from build123d import *

# Parameters (mm, degrees)
RECTANGLE127_AS_DRAWN_W                      = 25
RECTANGLE127_AS_DRAWN_H                      = 3
EXTRUDE155_DEPTH                             = 3
EXTRUDE155_ONTO_RECTANGLE127_ROLL_ANGLE      = -90
EXTRUDE155_ONTO_RECTANGLE127_PLACEMENT_ANGLE = 180
RECTANGLE128_AS_DRAWN_W                      = 25
RECTANGLE128_AS_DRAWN_H                      = 3
EXTRUDE157_DEPTH                             = 3
EXTRUDE157_ONTO_RECTANGLE128_ROLL_ANGLE      = -90
EXTRUDE157_ONTO_RECTANGLE128_PLACEMENT_ANGLE = 180
RECTANGLE130_AS_DRAWN_W                      = 25
RECTANGLE130_AS_DRAWN_H                      = 3
EXTRUDE162_DEPTH                             = 3
EXTRUDE162_ONTO_RECTANGLE130_ROLL_ANGLE      = -90
EXTRUDE162_ONTO_RECTANGLE130_PLACEMENT_ANGLE = 180
EXTRUDE160_DEPTH                             = 3
EXTRUDE160_ONTO_RECTANGLE127_ROLL_ANGLE      = -90
EXTRUDE160_ONTO_RECTANGLE127_PLACEMENT_ANGLE = 180
RECTANGLE132_AS_DRAWN_W                      = 3
RECTANGLE132_AS_DRAWN_H                      = 19.5
EXTRUDE168_DEPTH                             = 3
EXTRUDE168_ONTO_RECTANGLE132_ROLL_ANGLE      = -90
EXTRUDE168_ONTO_RECTANGLE132_PLACEMENT_ANGLE = 180
BOX043_W                                     = 100
BOX043_H                                     = 3
BOX043_DEPTH                                 = 45


with BuildPart() as extrude155:
    # Rectangle127 as drawn → Extrude155 (new)
    with BuildSketch(Plane.XY):
        with Locations((12.5, 1.5)):
            Rectangle(RECTANGLE127_AS_DRAWN_W, RECTANGLE127_AS_DRAWN_H)
    extrude(amount=-EXTRUDE155_DEPTH)


with BuildPart() as extrude155_1:
    # Extrude155 onto Rectangle127 roll: moved
    add(extrude155.part.rotate(Axis((0, 0, 0), (1, 0, 0)), EXTRUDE155_ONTO_RECTANGLE127_ROLL_ANGLE))


with BuildPart() as extrude155_2:
    # Extrude155 onto Rectangle127 placement: moved
    add(extrude155_1.part.moved(Location((114, -77, -70))).rotate(Axis((114, -77, -70), (0, 0, 1)), EXTRUDE155_ONTO_RECTANGLE127_PLACEMENT_ANGLE))


with BuildPart() as extrude155_3:
    # Extrude155 placement: moved
    add(extrude155_2.part.moved(Location((-183, 0, 0))))


with BuildPart() as extrude157:
    # Rectangle128 as drawn → Extrude157 (new)
    with BuildSketch(Plane.XY):
        with Locations((12.5, 1.5)):
            Rectangle(RECTANGLE128_AS_DRAWN_W, RECTANGLE128_AS_DRAWN_H)
    extrude(amount=-EXTRUDE157_DEPTH)


with BuildPart() as extrude157_1:
    # Extrude157 onto Rectangle128 roll: moved
    add(extrude157.part.rotate(Axis((0, 0, 0), (1, 0, 0)), EXTRUDE157_ONTO_RECTANGLE128_ROLL_ANGLE))


with BuildPart() as extrude157_2:
    # Extrude157 onto Rectangle128 placement: moved
    add(extrude157_1.part.moved(Location((89, -77, -70))).rotate(Axis((89, -77, -70), (0, 0, 1)), EXTRUDE157_ONTO_RECTANGLE128_PLACEMENT_ANGLE))


with BuildPart() as extrude157_3:
    # Extrude157 placement: moved
    add(extrude157_2.part.moved(Location((-208, 0, 0))))


with BuildPart() as extrude162:
    # Rectangle130 as drawn → Extrude162 (new)
    with BuildSketch(Plane.XY):
        with Locations((12.5, 1.5)):
            Rectangle(RECTANGLE130_AS_DRAWN_W, RECTANGLE130_AS_DRAWN_H)
    extrude(amount=-EXTRUDE162_DEPTH)


with BuildPart() as extrude162_1:
    # Extrude162 onto Rectangle130 roll: moved
    add(extrude162.part.rotate(Axis((0, 0, 0), (1, 0, 0)), EXTRUDE162_ONTO_RECTANGLE130_ROLL_ANGLE))


with BuildPart() as extrude162_2:
    # Extrude162 onto Rectangle130 placement: moved
    add(extrude162_1.part.moved(Location((39, -77, -70))).rotate(Axis((39, -77, -70), (0, 0, 1)), EXTRUDE162_ONTO_RECTANGLE130_PLACEMENT_ANGLE))


with BuildPart() as extrude162_3:
    # Extrude162 placement: moved
    add(extrude162_2.part.moved(Location((-183, 0, -42))))


with BuildPart() as extrude160:
    # Rectangle127 as drawn → Extrude160 (new)
    with BuildSketch(Plane.XY):
        with Locations((12.5, 1.5)):
            Rectangle(RECTANGLE127_AS_DRAWN_W, RECTANGLE127_AS_DRAWN_H)
    extrude(amount=-EXTRUDE160_DEPTH)


with BuildPart() as extrude160_1:
    # Extrude160 onto Rectangle127 roll: moved
    add(extrude160.part.rotate(Axis((0, 0, 0), (1, 0, 0)), EXTRUDE160_ONTO_RECTANGLE127_ROLL_ANGLE))


with BuildPart() as extrude160_2:
    # Extrude160 onto Rectangle127 placement: moved
    add(extrude160_1.part.moved(Location((114, -77, -70))).rotate(Axis((114, -77, -70), (0, 0, 1)), EXTRUDE160_ONTO_RECTANGLE127_PLACEMENT_ANGLE))


with BuildPart() as extrude160_3:
    # Extrude160 placement: moved
    add(extrude160_2.part.moved(Location((-208, 0, -42))))


with BuildPart() as fusion064027:
    # Rectangle132 as drawn → Extrude168 (new)
    with BuildSketch(Plane.XY):
        with Locations((1.5, 9.75)):
            Rectangle(RECTANGLE132_AS_DRAWN_W, RECTANGLE132_AS_DRAWN_H)
    extrude(amount=-EXTRUDE168_DEPTH)


with BuildPart() as fusion064027_1:
    # Extrude168 onto Rectangle132 roll: moved
    add(fusion064027.part.rotate(Axis((0, 0, 0), (1, 0, 0)), EXTRUDE168_ONTO_RECTANGLE132_ROLL_ANGLE))


with BuildPart() as fusion064027_2:
    # Extrude168 onto Rectangle132 placement: moved
    add(fusion064027_1.part.moved(Location((114, -77, -92.5))).rotate(Axis((114, -77, -92.5), (0, 0, 1)), EXTRUDE168_ONTO_RECTANGLE132_PLACEMENT_ANGLE))


with BuildPart() as fusion064027_3:
    # Extrude168 placement: moved
    add(fusion064027_2.part.moved(Location((-280, 0, 19.5))))

    # Fusion064027: union Extrude155, Extrude157, Extrude162, Extrude160
    add(extrude155_3.part)
    add(extrude157_3.part)
    add(extrude162_3.part)
    add(extrude160_3.part)


with BuildPart() as fusion064027_4:
    # Fusion064027 placement: moved
    add(fusion064027_3.part.moved(Location((0, 152, 0))))


with BuildPart() as cut035016:
    # Box043 → Box043 (new body)
    with BuildSketch(Plane(origin=(-169, 75, -115), x_dir=(1, 0, 0), z_dir=(0, 0, 1))):
        with Locations((50, 1.5)):
            Rectangle(BOX043_W, BOX043_H)
    extrude(amount=BOX043_DEPTH)

    # Cut035016: cut Fusion064027
    add(fusion064027_4.part, mode=Mode.SUBTRACT)


solid = cut035016.part
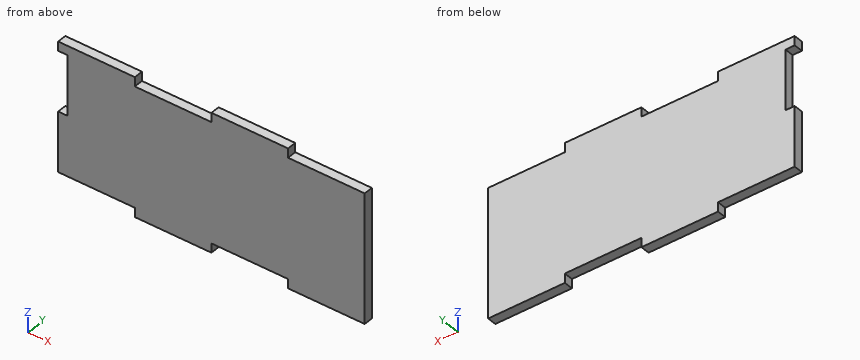
Verification items for the finished model (mm, model axes). Give positions to 0.01 mm unless a question says otherwise; leave off trailing zeros. Loops run counter-clockwise (first coordinate to the right, second up) from the corner with the lowest first, then second, coordinate; pieces in that order, holes last.
1. Cross-section at B-B on z = -88. Record the cut outline in (x, y).
Derived:
outline: (-166, 75) - (-69, 75) - (-69, 78) - (-166, 78) - close
2. Go/stop test with flat-tipped pins: P1, Ø0.9, axis at y = 76, z = -71, coming from the +X side; P2, Ø1.5, axis at x = -103.5, y = 76.5, coming from the -Z side; P3, Ø0.9, axis at y = 76, z = -113, coming from the -X side. Record where each tip stops, or that it passes through.
Derived:
P1: stops at x = -94
P2: stops at z = -112
P3: stops at x = -144
3. Cross-section at A-A on y = 77.45. Record the cut outline in (x, z), and give its area (3 significant figures).
Derived:
outline: (-169, -112) - (-144, -112) - (-144, -115) - (-119, -115) - (-119, -112) - (-94, -112) - (-94, -115) - (-69, -115) - (-69, -73) - (-94, -73) - (-94, -70) - (-119, -70) - (-119, -73) - (-144, -73) - (-144, -70) - (-169, -70) - (-169, -73) - (-166, -73) - (-166, -92.5) - (-169, -92.5) - close
area: 4,140 mm2
4. Material ranges on probe 1 along X at (y, z) = (76, -75.5); probe 2 along Z at (x, y) = (-82, 77.3); probe 3 along Z at (x, y) = (-159.5, 77.85), recorded low to high.
Derived:
probe 1: x = -166 to -69
probe 2: z = -115 to -73
probe 3: z = -112 to -70
5. Cross-section at C-C on x = -93. Record the cut outline in (y, z).
Derived:
outline: (75, -115) - (78, -115) - (78, -73) - (75, -73) - close
